from build123d import *

# Parameters (mm, degrees)
BOSS_EXTRUDE1_DEPTH = 3.175
SKETCH2_R           = 1.5875
SKETCH2_W           = 80.264
SKETCH2_H           = 12.954
CUT_EXTRUDE1_DEPTH  = 223.985606318
SKETCH7_R           = 1.5875
SKETCH7_W           = 46.99
SKETCH7_H           = 138.43
CUT_EXTRUDE4_DEPTH  = 223.985606318
CUT_EXTRUDE5_DEPTH  = 223.985606318
CUT_EXTRUDE8_DEPTH  = 221.482742149
SKETCH10_W          = 220.910927054
SKETCH10_H          = 122.260722121
CUT_EXTRUDE9_DEPTH  = 151.553414525


with BuildPart() as part:
    # Sketch1 → Boss-Extrude1 (new body)
    with BuildSketch(Plane(origin=(0, 0, 0), x_dir=(1, 0, 0), z_dir=(0, 1, 0))):
        with BuildLine():
            Line((-80, 112.5), (100, 112.5))
            Line((100, 112.5), (100, -112.5))
            Line((100, -112.5), (-80, -112.5))
            ThreePointArc((-80, -112.5), (-192.5, 0), (-80, 112.5))
        make_face()
    extrude(amount=-BOSS_EXTRUDE1_DEPTH)

    # Sketch2 → Cut-Extrude1 (cut, through all)
    with BuildSketch(Plane(origin=(0, 0, 0), x_dir=(1, 0, 0), z_dir=(0, 1, 0))):
        with Locations(Location((36.144045702, -74.2188, 0), (0, 0, 270))):
            Circle(SKETCH2_R)
        with Locations(Location((36.144045702, -67.8688, 0), (0, 0, 270))):
            Circle(SKETCH2_R)
        with Locations(Location((36.144045702, -61.5188, 0), (0, 0, 270))):
            Circle(SKETCH2_R)
        with Locations(Location((36.144045702, -55.1688, 0), (0, 0, 270))):
            Circle(SKETCH2_R)
        with Locations(Location((36.144045702, -48.8188, 0), (0, 0, 270))):
            Circle(SKETCH2_R)
        with Locations(Location((36.144045702, -42.4688, 0), (0, 0, 270))):
            Circle(SKETCH2_R)
        with Locations(Location((36.144045702, -36.1188, 0), (0, 0, 270))):
            Circle(SKETCH2_R)
        with Locations(Location((67.894045702, -74.2188, 0), (0, 0, 270))):
            Circle(SKETCH2_R)
        with Locations(Location((67.894045702, -67.8688, 0), (0, 0, 270))):
            Circle(SKETCH2_R)
        with Locations(Location((67.894045702, -61.5188, 0), (0, 0, 270))):
            Circle(SKETCH2_R)
        with Locations(Location((67.894045702, -55.1688, 0), (0, 0, 270))):
            Circle(SKETCH2_R)
        with Locations(Location((67.894045702, -48.8188, 0), (0, 0, 270))):
            Circle(SKETCH2_R)
        with Locations(Location((67.894045702, -42.4688, 0), (0, 0, 270))):
            Circle(SKETCH2_R)
        with Locations(Location((67.894045702, -36.1188, 0), (0, 0, 270))):
            Circle(SKETCH2_R)
        with Locations(Location((36.144045702, 74.2188, 0), (0, 0, 270))):
            Circle(SKETCH2_R)
        with Locations(Location((36.144045702, 67.8688, 0), (0, 0, 270))):
            Circle(SKETCH2_R)
        with Locations(Location((36.144045702, 61.5188, 0), (0, 0, 270))):
            Circle(SKETCH2_R)
        with Locations(Location((36.144045702, 55.1688, 0), (0, 0, 270))):
            Circle(SKETCH2_R)
        with Locations(Location((36.144045702, 48.8188, 0), (0, 0, 270))):
            Circle(SKETCH2_R)
        with Locations(Location((36.144045702, 42.4688, 0), (0, 0, 270))):
            Circle(SKETCH2_R)
        with Locations(Location((36.144045702, 36.1188, 0), (0, 0, 270))):
            Circle(SKETCH2_R)
        with Locations(Location((67.894045702, 74.2188, 0), (0, 0, 270))):
            Circle(SKETCH2_R)
        with Locations(Location((67.894045702, 67.8688, 0), (0, 0, 270))):
            Circle(SKETCH2_R)
        with Locations(Location((67.894045702, 61.5188, 0), (0, 0, 270))):
            Circle(SKETCH2_R)
        with Locations(Location((67.894045702, 55.1688, 0), (0, 0, 270))):
            Circle(SKETCH2_R)
        with Locations(Location((67.894045702, 48.8188, 0), (0, 0, 270))):
            Circle(SKETCH2_R)
        with Locations(Location((67.894045702, 42.4688, 0), (0, 0, 270))):
            Circle(SKETCH2_R)
        with Locations(Location((67.894045702, 36.1188, 0), (0, 0, 270))):
            Circle(SKETCH2_R)
        with Locations((52.019045702, -96.4438)):
            Rectangle(SKETCH2_W, SKETCH2_H)
        with Locations((52.019045702, 96.4438)):
            Rectangle(SKETCH2_W, SKETCH2_H)
    extrude(amount=-CUT_EXTRUDE1_DEPTH, mode=Mode.SUBTRACT)

    # Sketch7 → Cut-Extrude4 (cut, through all)
    with BuildSketch(Plane(origin=(0, 0, 0), x_dir=(1, 0, 0), z_dir=(0, 1, 0))):
        with Locations(Location((-50.166143469, 0, 0), (0, 0, 270))):
            Circle(SKETCH7_R)
        with Locations(Location((25.582761582, 0, 0), (0, 0, 270))):
            Circle(SKETCH7_R)
        with Locations(Location((87.462148806, 0, 0), (0, 0, 270))):
            Circle(SKETCH7_R)
        with Locations((-13.971143469, 0)):
            Rectangle(SKETCH7_W, SKETCH7_H)
    extrude(amount=-CUT_EXTRUDE4_DEPTH, mode=Mode.SUBTRACT)

    # Sketch8 → Cut-Extrude5 (cut, through all)
    with BuildSketch(Plane(origin=(0, 0, 0), x_dir=(1, 0, 0), z_dir=(0, 1, 0))):
        with BuildLine():
            Line((-167.0966, 25.4), (-229.776686608, 25.4))
            Line((-229.776686608, 25.4), (-229.776686608, -25.4))
            Line((-229.776686608, -25.4), (-167.0966, -25.4))
            ThreePointArc((-167.0966, -25.4), (-141.6966, 0), (-167.0966, 25.4))
        make_face()
    extrude(amount=-CUT_EXTRUDE5_DEPTH, mode=Mode.SUBTRACT)

    # Sketch9 → Cut-Extrude8 (cut, through all)
    with BuildSketch(Plane(origin=(0, 0, 0), x_dir=(1, 0, 0), z_dir=(0, 1, 0))):
        Polygon((-202.496068311, 81.375621875), (-202.496068311, 118.60629855), (0, 118.60629855), (0, 81.375621875), (22.483592167, 81.375621875), (22.483592167, -78.716287827), (0, -78.716287827), (0, -122.329366217), (-202.496068311, -122.329366217), (-202.496068311, -78.716287827), align=None)
    extrude(amount=-CUT_EXTRUDE8_DEPTH, mode=Mode.SUBTRACT)

    # Sketch10 → Cut-Extrude9 (cut, through all)
    with BuildSketch(Plane(origin=(0, 0, 0), x_dir=(1, 0, 0), z_dir=(0, 1, 0))):
        with Locations((38.526909819, -79.409861337)):
            Rectangle(SKETCH10_W, SKETCH10_H)
    extrude(amount=-CUT_EXTRUDE9_DEPTH, mode=Mode.SUBTRACT)


solid = part.part
Design review of the part built by this model. Coordinates are the model's own, in mm. A direction names the side the tool comes from. Give positions to 0.01 mm unless a question says otherwise; leave off trailing zeros. Loops run counter-clockwise (first coordinate to the right, second up) from the corner with the lowest first, then second, coordinate; pieces in that order, holes last. Notation, with made-up numbers: (53, -24.75) - (91, -24.75) arc R24 cw to (91, 5.25) - close; hole circle Ø8 at (88.5, 1). An arc over 180 degrees is marked (long way). Write item = value, one per line.
1) Take a section at C-C on z = -26. State the section outline as (x, y) points (3 decimals), and give its area (3 significant figures).
Result sheet:
outline = (22.484, -3.175) - (100, -3.175) - (100, 0) - (22.484, 0) - close
area = 246 mm2
2) To check wall thickness, follow line 1 (Z direction, x = 76, y = -2.35); line 2 (Z direction, x = 25.5, y = -1.8); line 3 (X direction, y = -1.7, z = -35.5). State the ranges of each line that lie inside material, in increasing order.
Result sheet:
line_1 = -112.5 to -102.92, -89.97 to 18.28
line_2 = -112.5 to -102.92, -89.97 to -1.59, 1.59 to 18.28
line_3 = 22.48 to 34.68, 37.61 to 66.43, 69.36 to 100
3) Draft analysis for pull direction Z (two halves, no side actions). For faces 4 (the face through (11, -2, -81.376)), 5 (the face through (62, 0, -48)), 6 (the face through (36.214, -1.565, -75.805)), 7 (the face through (36.214, -1.565, -63.105)), state which applies: +Z half, -Z half, draft (parallel to the pull), parting line (faces both ways), or undercut.
Result sheet:
face_4 = +Z half
face_5 = draft
face_6 = undercut
face_7 = undercut
4) Take a section at A-A on z = 0. State the section outline as (x, y) points (3 decimals).
Result sheet:
outline = (22.484, -3.175) - (23.995, -3.175) - (23.995, 0) - (22.484, 0) - close; (27.17, -3.175) - (85.875, -3.175) - (85.875, 0) - (27.17, 0) - close; (89.05, -3.175) - (100, -3.175) - (100, 0) - (89.05, 0) - close
5) Take a section at B-B on y = -0.8. Count the separate pieces of the cut face and the enclosed holes in it, and give its area (3 significant figures).
Result sheet:
separate_pieces = 1
enclosed_holes = 17
area = 9,670 mm2
6) Tool access review of faces 1 (the face through (22.484, -2, -32)), 2 (the face through (92.151, -2, -96)), 3 (the face through (0, -2, -97)): name each direction out of +Z, -Z, +X, -X, +Y, -Y from which nothing blocks a thin tool from reaching the whole face with its end or side.
Result sheet:
face_1 = +Z, -X, +Y, -Y
face_2 = +Y, -Y
face_3 = +Z, -Z, -X, +Y, -Y
7) Clearance check with a flat-ended pin moving along its axis: pin 1 Ø2.5 at (x, z) = (67.89, -61.52) entering from -Y. State where the tip first meets the part, or that it passes through.
Result sheet:
pin_1 = through
